The listing builds one solid part. Answer for the finished solid, in the listing's coordinates (mm). A direction names the side the tool comes from. Coordinates: 2 decimals unless noted, no trailing zeros. Write each loop counter-clockwise with the first axis right and the second up, starting at its lowest first coordinate (ties: lowest second). Pieces come first, ordered by that corner, then holes. Notation, with made-up numbers: M 29.25,70 L 63.25,70 A25 cw 63.25,94 Z; hole C 41.5,1 d9. An arc over 180 degrees is marked long. Answer as a JSON object with one key per item and string values. Group by question number.
from build123d import *

# Parameters (mm, degrees)
CROQUIS1_R              = 13.05
SALIENTE_EXTRUIR1_DEPTH = 35
REDONDEO1_R             = 10
REDONDEO2_R             = 5
CROQUIS2_R              = 2.05
CORTAR_EXTRUIR1_DEPTH   = 85.749277283


with BuildPart() as part:
    # Croquis1 → Saliente-Extruir1 (new body)
    with BuildSketch(Plane.XY):
        with BuildLine():
            Line((-20, 2.5), (-20, 41.3))
            ThreePointArc((-20, 41.3), (0, 61.3), (20, 41.3))
            Line((20, 41.3), (20, 2.5))
            Line((20, 2.5), (50, 2.5))
            Line((50, 2.5), (50, -2.5))
            Line((50, -2.5), (-50, -2.5))
            Line((-50, -2.5), (-50, 2.5))
            Line((-50, 2.5), (-20, 2.5))
        make_face()
        with Locations((0, 41.3)):
            Circle(CROQUIS1_R, mode=Mode.SUBTRACT)
    extrude(amount=SALIENTE_EXTRUIR1_DEPTH)

    # Redondeo1
    redondeo1_edges = [part.edges().sort_by_distance(p)[0] for p in [
        (20, 2.5, 17.5),
        (-20, 2.5, 17.5),
    ]]
    fillet(redondeo1_edges, radius=REDONDEO1_R)

    # Redondeo2
    redondeo2_edges = [part.edges().sort_by_distance(p)[0] for p in [
        (50, 0, 0),
        (-50, 0, 0),
        (-50, 0, 35),
        (50, 0, 35),
    ]]
    fillet(redondeo2_edges, radius=REDONDEO2_R)

    # Croquis2 → Cortar-Extruir1 (cut, through all)
    with BuildSketch(Plane(origin=(0, 2.5, 0), x_dir=(1, 0, 0), z_dir=(0, 1, 0))):
        with Locations(Location((-40, -17.5, 0), (0, 0, 270))):
            Circle(CROQUIS2_R)
        with Locations(Location((40, -17.5, 0), (0, 0, 90))):
            Circle(CROQUIS2_R)
    extrude(amount=-CORTAR_EXTRUIR1_DEPTH, mode=Mode.SUBTRACT)


solid = part.part
Item 1: A cutting plane is placed at B-B, the plane z = 17.5. Write down the section's boundary in (x, y), and give its area (3 significant figures).
Item 2: A tool of negligible diameter and unlimited length cuts with its end or side. For faces 5 (the face through (-20, 27, 17)), 6 (the face through (20, 27, 17)), 7 (the face through (1, -2.5, 17)), from which of +Z, -Z, +X, -X, +Y, -Y can it reach the whole face along a straight path? Write none if from no direction.
Item 3: A cutting plane is placed at A-A, the plane x = -40. Write down the section's boundary in (y, z).
Item 4: For a pull along X with two mould halves and no side action, classify faces 1 (the face through (50, 0, 17)), 2 (the face through (1, 23, 35)), 3 (the face through (37.967, 0.035, 17.767)), 4 (the face through (-48, 0, 34)) as +X half, -X half, draft (parallel to the pull), parting line (faces both ways), or undercut.
Item 5: Flat-ended cylindrical pins translate along their axes: pin 1 Ø12 at (y, z) = (31.5, 10) entering from -X; pin 2 Ø1 at (y, z) = (53.5, 15.5) entering from -X; pin 3 Ø1.5 at (x, z) = (-24, 15) entering from +Y. Find the tip coordinate at first contact, or state that the pin passes through.
Item 6: A cutting plane is placed at C-C, the plane z = 12.5. Write down the section's boundary in (x, y).
Item 7: Consider L1, parallel to X at y = -0.15, z = 17.5; L2, parallel to Y at x = 0, z = 19.5; L3, parallel to Z at x = 40, y = -0.95. Determine where each line is inside the solid, lowest interval first. Write a range as from..to.
Item 8: A cutting plane is placed at D-D, the plane y = 36. Write down the section's boundary in (x, z).
Answer:
{
 "1": {"outline": "M -50,-2.5 L -42.05,-2.5 L -42.05,2.5 L -50,2.5 Z; M -37.95,-2.5 L 37.95,-2.5 L 37.95,2.5 L 30,2.5 A10 cw 20,12.5 L 20,41.3 A20 ccw -20,41.3 L -20,12.5 A10 cw -30,2.5 L -37.95,2.5 Z; M 42.05,-2.5 L 50,-2.5 L 50,2.5 L 42.05,2.5 Z; hole C 0,41.3 d26.1", "area": "2,150 mm2"},
 "2": {"face 5": "+Z, -Z, -X, +Y", "face 6": "+Z, -Z, +X, +Y", "face 7": "+Z, -Z, +X, -X, -Y"},
 "3": {"outline": "M -2.5,0 L 2.5,0 L 2.5,15.45 L -2.5,15.45 Z; M -2.5,19.55 L 2.5,19.55 L 2.5,35 L -2.5,35 Z"},
 "4": {"face 1": "+X half", "face 2": "draft", "face 3": "undercut", "face 4": "-X half"},
 "5": {"pin 1": "x = -20", "pin 2": "x = -16.22", "pin 3": "y = 5.12"},
 "6": {"outline": "M -50,-2.5 L 50,-2.5 L 50,2.5 L 30,2.5 A10 cw 20,12.5 L 20,41.3 A20 ccw -20,41.3 L -20,12.5 A10 cw -30,2.5 L -50,2.5 Z; hole C 0,41.3 d26.1"},
 "7": {"L1": "-50..-42.05, -37.95..37.95, 42.05..50", "L2": "-2.5..28.25, 54.35..61.3", "L3": "0..15.45, 19.55..35"},
 "8": {"outline": "M -20,0 L -11.93,0 L -11.93,35 L -20,35 Z; M 11.93,0 L 20,0 L 20,35 L 11.93,35 Z"}
}
